Here's how the part is built. I have some questions about the finished solid (model axes, mm). Face numbers are marked on the shaded views. A direction names the side the tool comes from. Round coordinates to 2 decimals unless told otherwise and drop trailing zeros. Write each loop counter-clockwise with the first axis right and the second up, starting at its lowest first coordinate (ties: lowest second). Pieces come first, ordered by that corner, then holes. Notation, with made-up numbers: M 46.25,51 L 87.25,51 A20 ccw 87.25,90 Z; hole C 11.5,38 d2. An arc over 180 degrees is marked long. Use one line per item in the form item = value. Start each with the question number.
Q1. For the marked faces 1, 2 and 3, which set-ups out of +Z, -Z, +X, -X, +Y, -Y let a thin tool reach every point of the face, with its end or its side?
Q2. I need wall thicknesses on line 1 along X through (y, z) = (9.25, 5.4); line 2 along Z through (x, y) = (1.55, 10.5); line 3 along Y through (x, z) = (1.3, 3.65). Which ranges of each line are inside material? Lowest first, please. Write a range as from..to.
Q3. I want a section at A-A on y = 11.25. List the corners of the cut face in (x, z) for me, and give its area (3 significant figures).
Q4. I want a section at B-B on x = 1. List the corners of the cut face in (y, z) for me.
Q5. I want a section at C-C on y = 12.5. List the corners of the cut face in (x, z) for me.
Q6. I want a section at D-D on z = 2.7. List the corners of the cut face in (x, y) for me.
Q7. I'm going to push flat-ended pins straight in: pin 1 Ø2 at (y, z) = (4.5, 3) entering from -X; pin 2 Ø1.5 at (x, y) = (3.5, 5) entering from -Z; pin 3 Ø1.5 at (x, y) = (1, 9.5) entering from -Z. Where does each tip first touch, or does it pass through?
Q8. We'd pull the mould along X, two halves only. Please class the marked faces 4, 5, 6 and 7: +X half, -X half, draft (parallel to the pull), parting line (faces both ways), or undercut.
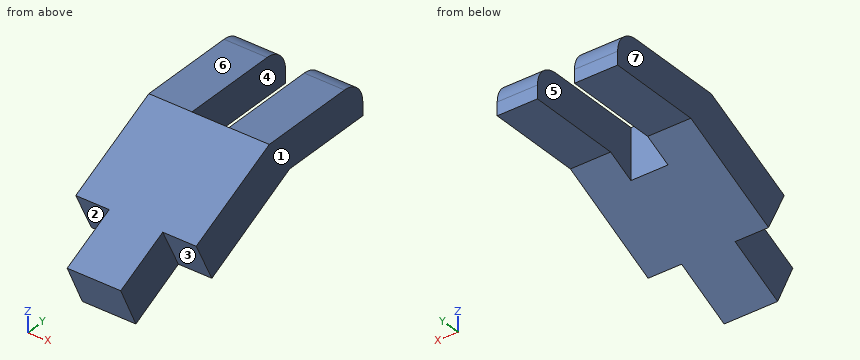
```python
from build123d import *

# Parameters (mm, degrees)
BOSS_EXTRUDE1_DEPTH            = 4.5
CUT_EXTRUDE1_REACH             = 3.412
SKETCH4_W                      = 1.385219638
SKETCH4_H                      = 4.6
CUT_EXTRUDE1_DIRECTION_2_DEPTH = 4.5
FILLET1_R                      = 0.9
CUT_EXTRUDE3_REACH             = 6.201
SKETCH9_W                      = 1.25
SKETCH9_H                      = 2.324916291


with BuildPart() as part:
    # Sketch3 → Boss-Extrude1 (new body)
    with BuildSketch(Plane(origin=(0, 0, 0), x_dir=(0, 0, -1), z_dir=(1, 0, 0))):
        Polygon((-5.191543854, 13.25823412), (-5.18615245, 9.674078564), (-2.262529631, 3.784549229), (-3.838080431, 3.04292615), (-6.584072535, 8.678891581), (-6.584072535, 13.25823412), align=None)
    extrude(amount=BOSS_EXTRUDE1_DEPTH)

    # Sketch4 → Cut-Extrude1 (cut, up to next)
    with BuildSketch(Plane(origin=(0, -0.010796619, 5.165911314), x_dir=(-1, 0, 0), z_dir=(0, 0.002089969, -0.999997816)), mode=Mode.PRIVATE) as cut_extrude1_sk1:
        with Locations((-2.304435674, 10.989683529)):
            Rectangle(SKETCH4_W, SKETCH4_H)
    cut_extrude1_tool1 = extrude(cut_extrude1_sk1.sketch, amount=-CUT_EXTRUDE1_REACH, mode=Mode.PRIVATE) & part.part
    add(cut_extrude1_tool1.solids().sort_by_distance((2.304436, 10.978863, 5.188879))[0], mode=Mode.SUBTRACT)

    # Sketch4 → Cut-Extrude1 direction 2 (cut)
    with BuildSketch(Plane(origin=(0, -0.010796619, 5.165911314), x_dir=(-1, 0, 0), z_dir=(0, 0.002089969, -0.999997816))):
        with Locations((-2.304435674, 10.989683529)):
            Rectangle(SKETCH4_W, SKETCH4_H)
    extrude(amount=CUT_EXTRUDE1_DIRECTION_2_DEPTH, mode=Mode.SUBTRACT)

    # Fillet1
    fillet1_edges = [part.edges().sort_by_distance(p)[0] for p in [
        (3.748522747, 13.25823412, 6.584072535),
        (0.805912927, 13.25823412, 6.584072535),
    ]]
    fillet(fillet1_edges, radius=FILLET1_R)

    # Sketch9 → Cut-Extrude3 (cut, up to next)
    with BuildSketch(Plane(origin=(0, -0.152871347, 0.307953638), x_dir=(-1, 0, 0), z_dir=(0, 0.444639458, -0.895709636)), mode=Mode.PRIVATE) as cut_extrude3_sk1:
        with Locations((-0.625, 5.558325308)):
            Rectangle(SKETCH9_W, SKETCH9_H)
    cut_extrude3_tool1 = extrude(cut_extrude3_sk1.sketch, amount=-CUT_EXTRUDE3_REACH, mode=Mode.PRIVATE) & part.part
    add(cut_extrude3_tool1.solids().sort_by_distance((0.625, 4.825774, 2.779404))[0], mode=Mode.SUBTRACT)
    # Sketch9 → Cut-Extrude3 (cut, up to next)
    with BuildSketch(Plane(origin=(0, -0.152871347, 0.307953638), x_dir=(-1, 0, 0), z_dir=(0, 0.444639458, -0.895709636)), mode=Mode.PRIVATE) as cut_extrude3_sk2:
        with Locations((-3.875, 5.558325308)):
            Rectangle(SKETCH9_W, SKETCH9_H)
    cut_extrude3_tool2 = extrude(cut_extrude3_sk2.sketch, amount=-CUT_EXTRUDE3_REACH, mode=Mode.PRIVATE) & part.part
    add(cut_extrude3_tool2.solids().sort_by_distance((3.875, 4.825774, 2.779404))[0], mode=Mode.SUBTRACT)


solid = part.part
```
Reported:
q1.face_1 = +Z, -Z, +X, +Y, -Y
q1.face_2 = -Z, -X, -Y
q1.face_3 = -Z, +X, -Y
q2.line_1 = 0..1.61, 3..4.5
q2.line_2 = 5.19..6.58
q2.line_3 = 3.13..6.58
q3.outline = M 0,5.19 L 1.61,5.19 L 1.61,6.58 L 0,6.58 Z; M 3,5.19 L 4.5,5.19 L 4.5,6.58 L 3,6.58 Z
q3.area = 4.35 mm^2
q4.outline = M 5.1,4.84 L 5.87,3.3 L 9.67,5.19 L 13.26,5.19 L 13.26,5.68 A0.9 ccw 12.36,6.58 L 8.68,6.58 Z
q5.outline = M 0,5.19 L 1.61,5.19 L 1.61,6.57 L 0,6.57 Z; M 3,5.19 L 4.5,5.19 L 4.5,6.57 L 3,6.57 Z
q6.outline = M 1.25,3.58 L 3.25,3.58 L 3.25,4.67 L 1.25,4.67 Z
q7.pin_1 = 1.25
q7.pin_2 = 2.51
q7.pin_3 = 4.73
q8.face_4 = undercut
q8.face_5 = undercut
q8.face_6 = draft
q8.face_7 = -X half
